```python
from build123d import *

# Parameters (mm, degrees)
F1_DEPTH      = 19.84375
F1_DEPTH_BACK = 19.84375
F2_START      = 17.30375
F2_DEPTH      = 2.54
F3_START      = -17.30375
F3_DEPTH      = 2.54
F4_R          = 159.2477786005
F4_R_2        = 133.35
F5_DEPTH      = 127


with BuildPart() as f1:
    # F0 (on Right) → F1 (new body, two sides)
    with BuildSketch(Plane.YZ) as f1_sk:
        Polygon((31.5376230345, 32.8083333333), (0, 0), (0, -3.6651832175), (35.060848841, 32.8083333333), align=None)
    extrude(amount=F1_DEPTH)
    extrude(f1_sk.sketch, amount=-F1_DEPTH_BACK)

    # F0 (on Right) → F2 (join)
    with BuildSketch(Plane.YZ.offset(F2_START)):
        Polygon((0, 32.8083333333), (0, 0), (31.5376230345, 32.8083333333), align=None)
    extrude(amount=F2_DEPTH)

    # F0 (on Right) → F3 (join)
    with BuildSketch(Plane.YZ.offset(F3_START)):
        Polygon((0, 32.8083333333), (0, 0), (31.5376230345, 32.8083333333), align=None)
    extrude(amount=-F3_DEPTH)

    # F4 (on Front) → F5 (cut)
    with BuildSketch(Plane.XZ):
        with Locations((0, -104.29066769)):
            Circle(F4_R)
        with Locations((0, -104.29066769)):
            Circle(F4_R_2, mode=Mode.SUBTRACT)
    extrude(amount=-F5_DEPTH, mode=Mode.SUBTRACT)


solid = f1.part
```
Here's how the part is built. I have some questions about the finished solid (model axes, mm). A direction names the side the tool comes from. Coordinates: 2 decimals unless noted, no trailing zeros. Order: outer loops, then holes, each group sorted by start corner. A loop starts at its lowest first (then second) coordinate and runs counter-clockwise, first axis right, second up. Notation, with made-up numbers: M 9,-18 L 41,-18 A26 cw 41,11 Z; hole C -27.75,24.25 d9. An arc over 180 degrees is marked long. Answer as a JSON object with one key per item and string values. Group by question number.
(1) Which directions (+Z, -Z, +X, -X, +Y, -Y) give clear straight access to the entire face, cutting with the end or side of a thin tool? Please do faces 1 (the face through (19.844, 11, 16)), 2 (the face through (0.24, 14.16, 14.73)).
(2) Suppose I cut it at C-C, the plane x = -5.5. Please give me the cut outline in (y, z).
(3) Suppose I cut it at D-D, the plane x = -0.5. Please give me the cut outline in (y, z).
(4) If we mould it in two halves opening along X, with no side actions, what happens to faces 3 (the face through (1.57, 28.73, 29.05)), 4 (the face through (-17.304, 10, 17)), 5 (the face through (2, 0, -1))? For each: released by +X, released by -X, zero draft, split by the parting line, or undercut.
(5) I need wall thicknesses on probe 1 along X at (y, z) = (11.5, 22.5); probe 2 along Z at (x, y) = (-10.5, 30); probe 3 along Z at (x, y) = (-15, 29). Which ranges of each line are inside material? Lowest first, please.
(6) Suppose I cut it at A-A, the plane y = 11.5. Please give me the cut outline in (x, z), then the cut area to 3 significant figures.
(7) For pin 1 (8 mm diameter, centred on x = -11, y = 13, fed in from +Z); pin 2 (1 mm diameter, centred on x = 15, z = 10.5, fed in from -Y); pin 3 (10 mm diameter, centred on x = 12.5, z = 12, fed in from +Y); pin 4 (5 mm diameter, centred on x = 12.5, z = 1, fed in from -Y), each with a flat end and sliding along its axis, tell me the tip position at first contact or that it passes through.
(8) Suppose I cut it at B-B, the plane z = 22.5. Please give me the cut outline in (x, y), then the cut area to 3 significant figures.
Values found:
{
 "1": {"face 1": "+Z, -Z, +X, +Y, -Y", "face 2": "+Z, -Y"},
 "2": {"outline": "M 0,-3.67 L 31.35,28.95 L 27.82,28.95 L 0,0 Z"},
 "3": {"outline": "M 0,-3.67 L 31.46,29.06 L 27.93,29.06 L 0,0 Z"},
 "4": {"face 3": "split by the parting line", "face 4": "undercut", "face 5": "zero draft"},
 "5": {"probe 1": "x = -19.84 to -17.3, 17.3 to 19.84", "probe 2": "z = 27.54 to 28.65", "probe 3": "z = 26.5 to 28.21"},
 "6": {"outline": "M -19.84,8.3 L 19.84,8.3 L 19.84,27.57 A133.35 ccw 17.3,27.93 L 17.3,11.96 L -17.3,11.96 L -17.3,27.93 A133.35 ccw -19.84,27.57 Z", "area": "226 mm^2"},
 "7": {"pin 1": "stops at z = 17.68", "pin 2": "stops at y = 9.61", "pin 3": "stops at y = 19.86", "pin 4": "stops at y = 0"},
 "8": {"outline": "M -19.84,0 L -17.3,0 L -17.3,21.63 L 17.3,21.63 L 17.3,0 L 19.84,0 L 19.84,25.15 L -19.84,25.15 Z", "area": "250 mm^2"}
}
